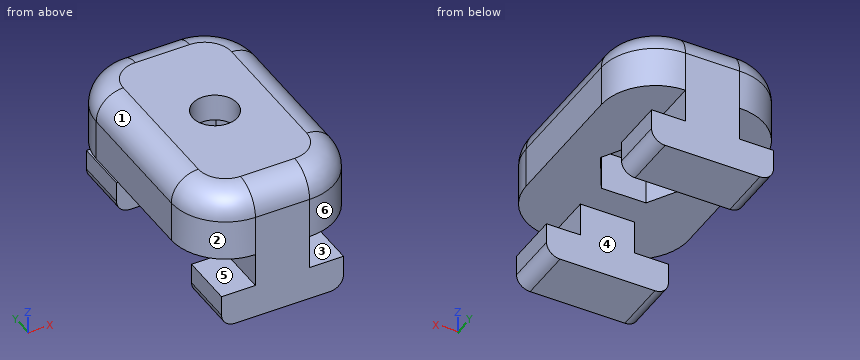
```python
from build123d import *

# Parameters (mm, degrees)
BOSS_EXTRU_3_DEPTH      = 4
ESQUISSE3_W             = 12
ESQUISSE3_H             = 5
BOSS_EXTRU_4_DEPTH      = 5
ENL_V_MAT_EXTRU_1_REACH = 7
ESQUISSE4_R             = 1.65
ENL_V_MAT_EXTRU_2_DEPTH = 3
CONG_1_R                = 4
CONG_2_R                = 2


with BuildPart() as part:
    # Esquisse2 → Boss.-Extru.3 (new body)
    with BuildSketch(Plane(origin=(0, 0, 0), x_dir=(1, 0, 0), z_dir=(0, 1, 0))):
        with BuildLine():
            Line((11.568725398, 38.128215269), (18.568725398, 38.128215269))
            ThreePointArc((18.568725398, 38.128215269), (19.275832179, 37.83532205), (19.568725398, 37.128215269))
            Line((19.568725398, 37.128215269), (19.568725398, 35.628215269))
            Line((19.568725398, 35.628215269), (17.068725398, 35.628215269))
            Line((17.068725398, 35.628215269), (17.068725398, 33.128215269))
            Line((17.068725398, 33.128215269), (21.068725398, 33.128215269))
            Line((21.068725398, 33.128215269), (21.068725398, 28.128215269))
            Line((21.068725398, 28.128215269), (9.068725398, 28.128215269))
            Line((9.068725398, 28.128215269), (9.068725398, 33.128215269))
            Line((9.068725398, 33.128215269), (13.068725398, 33.128215269))
            Line((13.068725398, 33.128215269), (13.068725398, 35.628215269))
            Line((13.068725398, 35.628215269), (10.568725398, 35.628215269))
            Line((10.568725398, 35.628215269), (10.568725398, 37.128215269))
            ThreePointArc((10.568725398, 37.128215269), (10.861618616, 37.83532205), (11.568725398, 38.128215269))
        make_face()
    extrude(amount=BOSS_EXTRU_3_DEPTH)

    # Esquisse3 → Boss.-Extru.4 (add)
    with BuildSketch(Plane(origin=(0, 4, 0), x_dir=(1, 0, 0), z_dir=(0, 1, 0))):
        with Locations((15.068725398, 30.628215269)):
            Rectangle(ESQUISSE3_W, ESQUISSE3_H)
    extrude(amount=BOSS_EXTRU_4_DEPTH)

    # Symétrie1: part across plane


with BuildPart() as part_1:
    add(part.part)
    add(part.part.mirror(Plane.ZX.offset(9)))

    # Esquisse4 → Enlèv. mat.-Extru.1 (cut, up to next)
    with BuildSketch(Plane(origin=(0, 0, -33.128215269), x_dir=(-1, 0, 0), z_dir=(0, 0, -1)), mode=Mode.PRIVATE) as enl_v_mat_extru_1_sk1:
        with Locations((-15.068725398, 9)):
            Circle(ESQUISSE4_R)
    enl_v_mat_extru_1_tool1 = extrude(enl_v_mat_extru_1_sk1.sketch, amount=-ENL_V_MAT_EXTRU_1_REACH, mode=Mode.PRIVATE) & part_1.part
    add(enl_v_mat_extru_1_tool1.solids().sort_by_distance((15.068725, 9, -33.128215))[0], mode=Mode.SUBTRACT)

    # Esquisse5 → Enlèv. mat.-Extru.2 (cut)
    with BuildSketch(Plane(origin=(0, 0, -33.128215269), x_dir=(-1, 0, 0), z_dir=(0, 0, -1))):
        Polygon((-13.42327713, 11.85), (-16.714173665, 11.85), (-18.359621932, 9), (-16.714173665, 6.15), (-13.42327713, 6.15), (-11.777828863, 9), align=None)
    extrude(amount=-ENL_V_MAT_EXTRU_2_DEPTH, mode=Mode.SUBTRACT)

    # Congé1
    cong_1_edges = [part_1.edges().sort_by_distance(p)[0] for p in [
        (9.068725398, 0, -30.628215269),
        (9.068725398, 18, -30.628215269),
        (21.068725398, 18, -30.628215269),
        (21.068725398, 0, -30.628215269),
    ]]
    fillet(cong_1_edges, radius=CONG_1_R)

    # Congé2
    cong_2_edges = [part_1.edges().sort_by_distance(p)[0] for p in [
        (9.068725398, 9, -28.128215269),
        (15.068725398, 0, -28.128215269),
        (21.068725398, 9, -28.128215269),
        (15.068725398, 18, -28.128215269),
        (19.897152522, 16.828427125, -28.128215269),
        (19.897152522, 1.171572875, -28.128215269),
        (10.240298273, 16.828427125, -28.128215269),
        (10.240298273, 1.171572875, -28.128215269),
    ]]
    fillet(cong_2_edges, radius=CONG_2_R)


solid = part_1.part
```
Model file for the job. Use its own axes, mm. Face numbers are marked on the shaded views. A direction names the side the tool comes from. Give positions to 0.01 mm unless a question says otherwise; leave off trailing zeros. Order: outer loops, then holes, each group sorted by start corner. A loop starts at its lowest first (then second) coordinate and runs counter-clockwise, first axis right, second up.
1) Saw through at C-C, the plane y = 7.75. Write the cut outline in (x, z), then the cut area to 3 significant figures.
2) Saw through at A-A, the plane z = -35. Write the cut outline in (x, y).
3) Pin check, flat tips, straight feed: pin 1 (1 mm diameter, centred on y = 15.5, z = -30.5, fed in from -X); pin 2 (0.8 mm diameter, centred on y = 1.5, z = -34.5, fed in from +X); pin 3 (1.6 mm diameter, centred on y = 1.5, z = -36.5, fed in from -X). Stop position of each tip, or through.
4) 3-axis set-ups, long thin cutter, end or side, ignore diameter. For the marked faces 4, 5 and 6: which of +Z, -Z, +X, -X, +Y, -Y reach the whole face in a straight line?
5) Mould opens along Z. For the marked faces 1, 2 and 3 say: +Z half, -Z half, draft (parallel to the pull), parting line (faces both ways), or undercut.
6) Saw through at D-D, the plane y = 12.5. Write the cut outline in (x, z).
7) Wall check: probe 1 along Y at (x, z) = (16.5, -36); probe 2 along Z at (x, y) = (15, 6); probe 3 along X at (y, z) = (2, -33.75). Give the ranges that are in metal, low to high.
8) Saw through at B-B, the plane x = 16.25. Write the cut outline in (y, z).
Computed:
1. outline: (9.07, -33.13) - (12.5, -33.13) - (12.5, -30.13) - (13.99, -30.13) - (13.99, -28.13) - (11.07, -28.13) arc R2 ccw to (9.07, -30.13) - close; (16.15, -30.13) - (17.64, -30.13) - (17.64, -33.13) - (21.07, -33.13) - (21.07, -30.13) arc R2 ccw to (19.07, -28.13) - (16.15, -28.13) - close
1. area: 38.6 mm2
2. outline: (13.07, 0) - (17.07, 0) - (17.07, 4) - (13.07, 4) - close; (13.07, 14) - (17.07, 14) - (17.07, 18) - (13.07, 18) - close
3. pin 1: stops at x = 9.2
3. pin 2: stops at x = 17.07
3. pin 3: stops at x = 10.57
4. face 4: -Z, +X, -X
4. face 5: -X, +Y, -Y
4. face 6: +Z, +X, -Y
5. face 1: +Z half
5. face 2: draft
5. face 3: undercut
6. outline: (9.07, -33.13) - (21.07, -33.13) - (21.07, -30.13) arc R2 ccw to (19.07, -28.13) - (11.07, -28.13) arc R2 ccw to (9.07, -30.13) - close
7. probe 1: y = 0 to 4, 14 to 18
7. probe 2: z = -33.13 to -28.13
7. probe 3: x = 13.07 to 17.07
8. outline: (0, -38.13) - (4, -38.13) - (4, -33.13) - (6.15, -33.13) - (6.15, -30.13) - (7.85, -30.13) - (7.85, -28.13) - (2, -28.13) arc R2 ccw to (0, -30.13) - close; (10.15, -30.13) - (11.85, -30.13) - (11.85, -33.13) - (14, -33.13) - (14, -38.13) - (18, -38.13) - (18, -30.13) arc R2 ccw to (16, -28.13) - (10.15, -28.13) - close
